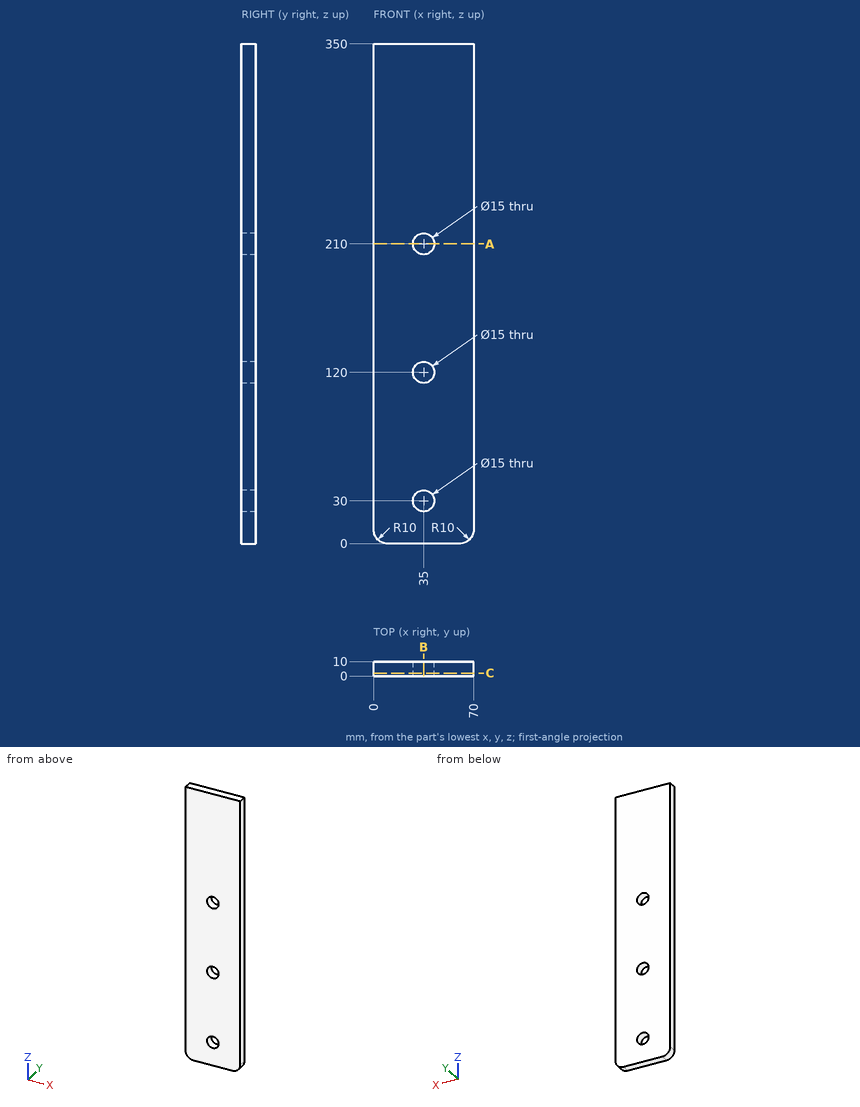
Here's the drawing with two shaded views (mm, measured from the low corner). I have some questions. Round coordinates to 2 decimals unless told otherwise and drop trailing zeros. Loops run counter-clockwise (first coordinate to the right, second up) from the corner with the lowest first, then second, coordinate; pieces in that order, holes last. Notation, with made-up numbers: M -30.75,-9 L -26.75,-9 A26 ccw -26.75,30 Z; hole C 65,-6.75 d4. An arc over 180 degrees is marked long. Put each result on its own line as item: value.
Q1. Imagine slicing it at C-C (y = 2). Write out the boundary of the cut face in (x, z).
Check result:
outline: M 0,10 A10 ccw 10,0 L 60,0 A10 ccw 70,10 L 70,350 L 0,350 Z; hole C 35,30 d15; hole C 35,120 d15; hole C 35,210 d15
Q2. For pin 1 (13.5 mm diameter, centred on x = 35, z = 210, fed in from -Y), with a flat end and sliding along its axis, tell me the tip position at first contact or that it passes through.
Check result:
pin 1: through
Q3. Imagine slicing it at A-A (z = 210). Write out the boundary of the cut face in (x, y).
Check result:
outline: M 0,0 L 27.5,0 L 27.5,10 L 0,10 Z; M 42.5,0 L 70,0 L 70,10 L 42.5,10 Z
Q4. I need wall thicknesses on probe 1 along Z at (x, y) = (35, 3.25); probe 2 along X at (y, z) = (5, 120); probe 3 along Z at (x, y) = (9, 7.5). Which ranges of each line are inside material? Lowest first, please.
Check result:
probe 1: 0 to 22.5, 37.5 to 112.5, 127.5 to 202.5, 217.5 to 350
probe 2: 0 to 27.5, 42.5 to 70
probe 3: 0.05 to 350
Q5. Imagine slicing it at B-B (x = 35). Write out the boundary of the cut face in (y, z).
Check result:
outline: M 0,0 L 10,0 L 10,22.5 L 0,22.5 Z; M 0,37.5 L 10,37.5 L 10,112.5 L 0,112.5 Z; M 0,127.5 L 10,127.5 L 10,202.5 L 0,202.5 Z; M 0,217.5 L 10,217.5 L 10,350 L 0,350 Z
